```python
from build123d import *

# Parameters (mm, degrees)
BOSS_EXTRUDE1_DEPTH = 9.8
SKETCH2_R           = 3.949999995
BOSS_EXTRUDE2_DEPTH = 1.2
SKETCH3_W           = 38.864651583
SKETCH3_H           = 1.2
CUT_EXTRUDE1_DEPTH  = 21.999977365
BOSS_EXTRUDE3_DEPTH = 2


with BuildPart() as part:
    # Sketch1 → Boss-Extrude1 (new body)
    with BuildSketch(Plane.XY.offset(11)):
        Polygon((4.333958961, -10.506317019), (10.493660346, -4.364516586), (10.506317019, 4.333958961), (4.364516586, 10.493660346), (-4.364516586, 10.493660346), (-10.506317019, 4.333958961), (-10.493660346, -4.364516586), (-4.333958961, -10.506317019), align=None)
        Polygon((0, 8.900009778), (3.673546249, 8.905354887), (8.894626983, 3.699447494), (8.905354887, -3.673546249), (3.699447494, -8.894626983), (0, -8.900009778), (-3.699447494, -8.894626983), (-8.905354887, -3.673546249), (-8.894626983, 3.699447494), (-3.673546249, 8.905354887), align=None, mode=Mode.SUBTRACT)
    extrude(amount=-BOSS_EXTRUDE1_DEPTH)

    # Sketch2 → Boss-Extrude2 (add)
    with BuildSketch(Plane(origin=(0, 0, 1.2), x_dir=(-1, 0, 0), z_dir=(0, 0, -1))):
        with BuildLine():
            Line((4.364516586, 10.493660346), (-4.364516586, 10.493660346))
            Line((-4.364516586, 10.493660346), (-10.506317019, 4.333958961))
            ThreePointArc((-10.506317019, 4.333958961), (-14.560364187, -0.021186842), (-10.493660346, -4.364516586))
            Line((-10.493660346, -4.364516586), (-4.333958961, -10.506317019))
            Line((-4.333958961, -10.506317019), (4.333958961, -10.506317019))
            Line((4.333958961, -10.506317019), (10.493660346, -4.364516586))
            ThreePointArc((10.493660346, -4.364516586), (14.560364187, -0.021186842), (10.506317019, 4.333958961))
            Line((10.506317019, 4.333958961), (4.364516586, 10.493660346))
        make_face()
        Circle(SKETCH2_R, mode=Mode.SUBTRACT)
    extrude(amount=BOSS_EXTRUDE2_DEPTH)

    # Sketch3 → Cut-Extrude1 (cut, through all)
    with BuildSketch(Plane.XZ.offset(10.506317019)):
        with Locations((0.864726488, 0.6)):
            Rectangle(SKETCH3_W, SKETCH3_H)
    extrude(amount=-CUT_EXTRUDE1_DEPTH, mode=Mode.SUBTRACT)

    # Sketch5 → Boss-Extrude3 (add)
    with BuildSketch(Plane(origin=(0, 0, 1.2), x_dir=(-1, 0, 0), z_dir=(0, 0, -1))):
        Polygon((-4.364516586, 10.493660346), (-10.506317019, 4.333958961), (-10.493660346, -4.364516586), (-4.333958961, -10.506317019), (4.333958961, -10.506317019), (10.493660346, -4.364516586), (10.506317019, 4.333958961), (4.364516586, 10.493660346), align=None)
        Polygon((-8.894626983, 3.699447494), (-8.905354887, -3.673546249), (-3.699447494, -8.894626983), (0, -8.900009778), (3.699447494, -8.894626983), (8.905354887, -3.673546249), (8.894626983, 3.699447494), (3.673546249, 8.905354887), (0, 8.900009778), (-3.673546249, 8.905354887), align=None, mode=Mode.SUBTRACT)
    extrude(amount=BOSS_EXTRUDE3_DEPTH)


solid = part.part
```
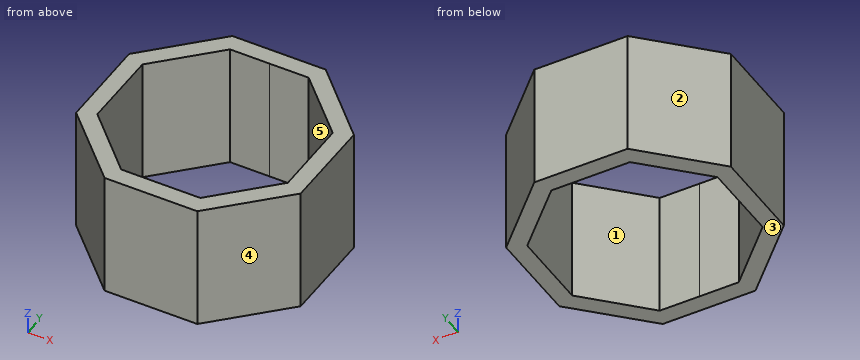
Input: part model. Units: mm. Frame: model coordinates. Face numbers are marked on the shaded views. A direction names the side the tool comes from. Coordinates: 2 decimals unless noted, no trailing zeros. Order: outer loops, then holes, each group sorted by start corner. A loop starts at its lowest first (then second) coordinate and runs counter-clockwise, first axis right, second up. Notation, with made-up numbers: (-20.75, 73.5) - (20.25, 73.5) arc R26 ccw to (20.25, 104.5) - close; hole circle Ø7 at (56.25, 22). An arc over 180 degrees is marked (long way). Put each result on its own line as item: value.
1. Contact query for flat-ended pins moving along their axis: pin 1 Ø1.5 at (y, z) = (1, 1) entering from +X; pin 2 Ø8 at (x, y) = (-0.5, 2) entering from -Z (1 decimal). Output: stop coordinate, or through.
Report:
pin 1: stops at x = 10.5
pin 2: passes through
2. Line query: line 1 along Y through (x, z) = (3.5, 6); line 2 along X through (y, z) = (-2.5, 3); line 3 along X through (y, z) = (6.25, 1.75). Output: solid intervals per line, ascending.
Report:
line 1: y = -10.51 to -8.89, 8.91 to 10.49
line 2: x = -10.5 to -8.9, 8.9 to 10.5
line 3: x = -8.6 to -6.34, 6.34 to 8.6
3. Cut plane B-B on x = 6. Return the cut outline in (y, z).
Report:
outline: (-8.85, -0.8) - (-6.59, -0.8) - (-6.59, 11) - (-8.85, 11) - close; (6.59, -0.8) - (8.85, -0.8) - (8.85, 11) - (6.59, 11) - close
4. Reachability of the marked faces 1 and 2 from +Z, -Z, +X, -X, +Y, -Y: full face, straight path, thin tool, end or side. Return the list, or none.
Report:
face 1: +Z, -Z
face 2: +Z, -Z, -X, +Y
5. Cut plane C-C on z = 5. Return the cut outline in (x, y).
Report:
outline: (-10.51, 4.33) - (-10.49, -4.36) - (-4.33, -10.51) - (4.33, -10.51) - (10.49, -4.36) - (10.51, 4.33) - (4.36, 10.49) - (-4.36, 10.49) - close; hole (-8.91, -3.67) - (-3.7, -8.89) - (0, -8.9) - (3.7, -8.89) - (8.91, -3.67) - (8.89, 3.7) - (3.67, 8.91) - (0, 8.9) - (-3.67, 8.91) - (-8.89, 3.7) - close
6. Cut plane A-A on y = -2.25. Return the cut outline in (x, z), then the cut area to 3 significant figures.
Report:
outline: (-10.5, -0.8) - (-8.9, -0.8) - (-8.9, 11) - (-10.5, 11) - close; (8.9, -0.8) - (10.5, -0.8) - (10.5, 11) - (8.9, 11) - close
area: 37.6 mm2
7. Draft query along X for the marked faces 3, 4 and 5. Return one class per face: pulls with the +X half, pulls with the -X half, needs draft (parallel to the pull), parting line crosses it, or undercut.
Report:
face 3: needs draft
face 4: pulls with the +X half
face 5: undercut
